For this review, take the finished solid that the model builds, in its own axes (mm). Face numbers are marked on the shaded views. A direction names the side the tool comes from. Give positions to 0.01 mm unless a question says otherwise; leave off trailing zeros. Order: outer loops, then holes, each group sorted by start corner. A loop starts at its lowest first (then second) coordinate and runs counter-clockwise, first axis right, second up. Notation, with made-up numbers: M 29,37.5 L 70,37.5 A23 ccw 70,63.5 Z; hole C -26.75,12 d4. An arc over 180 degrees is marked long. Answer as CSV lines item,"result". Start each with the question number.
1. Mouldability with a two-part tool opening along X and no side actions: class the marked faces 5, 6 and 7 as pulls with the +X half, pulls with the -X half, needs draft (parallel to the pull), parting line crosses it, or undercut.
2. We need section D-D, the plane x = -18. Give the boundary of the cut face in (y, z).
3. We need section B-B, the plane x = 4. Give the boundary of the cut face in (y, z).
4. Machinability: for the marked faces 1, 2, 3 and 4, which of the approach directions +Z, -Z, +X, -X, +Y, -Y give a long, thin tool a straight path to every point of the face, cutting with its end or side? Answer none if there is none.
5. For line 1 along X through (y, z) = (15, 4.25); line 2 along X through (y, z) = (3, 2.25); line 3 along X through (y, z) = (-26.5, 5.25), list the stretches that pass through material, from the lowest coordinate up.
6. Clearance check with flat-ended pins moving along their axes: P1, Ø5, axis at y = 1.5, z = 5.5, coming from the -X side; P2, Ø4.5, axis at y = 28, z = 3, coming from the +X side; P3, Ø3, axis at x = 35.5, z = 5, coming from the +Y side. State where each tip first meets the part, or that it passes through.
7. We need section A-A, the plane z = 7.5. Give the boundary of the cut face in (x, y).
8. We need section C-C, the plane y = 19. Give the boundary of the cut face in (x, z), and give its area (3 significant figures).
from build123d import *

# Parameters (mm, degrees)
EXTRUDE_1_DEPTH = 10


with BuildPart() as part:
    # 草图1 → 凸台-拉伸1 (new body)
    with BuildSketch(Plane.XY):
        Polygon((-28.32, 23.992), (-38.32, 23.992), (-38.32, 12.192), (-28.32, 12.192), (-28.32, -11.808), (-38.32, -11.808), (-38.32, -23.608), (-28.32, -23.608), (-28.32, -33.32), (28.32, -33.32), (38.32, -33.32), (38.32, -23.608), (28.32, -23.608), (28.32, 12.192), (38.32, 12.192), (38.32, 23.992), (28.32, 23.992), (28.32, 33.32), (-28.32, 33.32), align=None)
        Polygon((-20.065382953, 15.549088882), (13.215792231, -23.608), (-20.065382953, -23.608), align=None, mode=Mode.SUBTRACT)
        Polygon((19.961624404, -15.682069675), (-13.058637611, 23.695290925), (20.221802898, 23.474154822), align=None, mode=Mode.SUBTRACT)
    extrude(amount=EXTRUDE_1_DEPTH)


solid = part.part
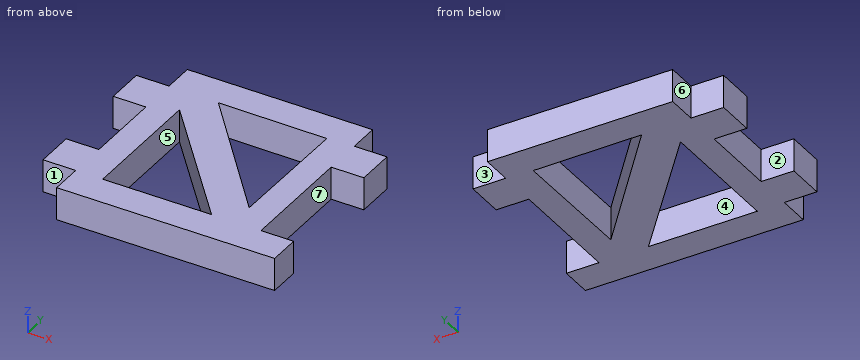
Result set:
1,face 5,"undercut"
1,face 6,"pulls with the -X half"
1,face 7,"pulls with the +X half"
2,outline,"M -33.32,0 L -23.61,0 L -23.61,10 L -33.32,10 Z; M 13.12,0 L 33.32,0 L 33.32,10 L 13.12,10 Z"
3,outline,"M -33.32,0 L -23.61,0 L -23.61,10 L -33.32,10 Z; M -12.77,0 L 3.35,0 L 3.35,10 L -12.77,10 Z; M 23.58,0 L 33.32,0 L 33.32,10 L 23.58,10 Z"
4,face 1,"+Z, -Z, -X, -Y"
4,face 2,"+Z, -Z, -X"
4,face 3,"+Z, -Z, +X, +Y"
4,face 4,"+Z, -Z"
5,line 1,"-38.32 to -20.07, -19.6 to -5.77, 20.17 to 38.32"
5,line 2,"-28.32 to -20.07, -9.4 to 4.3, 20.09 to 28.32"
5,line 3,"-28.32 to 38.32"
6,P1,"x = -28.32"
6,P2,"x = 28.32"
6,P3,"y = 23.99"
7,outline,"M -38.32,-23.61 L -28.32,-23.61 L -28.32,-33.32 L 38.32,-33.32 L 38.32,-23.61 L 28.32,-23.61 L 28.32,12.19 L 38.32,12.19 L 38.32,23.99 L 28.32,23.99 L 28.32,33.32 L -28.32,33.32 L -28.32,23.99 L -38.32,23.99 L -38.32,12.19 L -28.32,12.19 L -28.32,-11.81 L -38.32,-11.81 Z; hole M -20.07,-23.61 L 13.22,-23.61 L -20.07,15.55 Z; hole M -13.06,23.7 L 19.96,-15.68 L 20.22,23.47 Z"
8,outline,"M -38.32,0 L -9.12,0 L -9.12,10 L -38.32,10 Z; M 20.19,0 L 38.32,0 L 38.32,10 L 20.19,10 Z"
8,area,"473 mm2"
